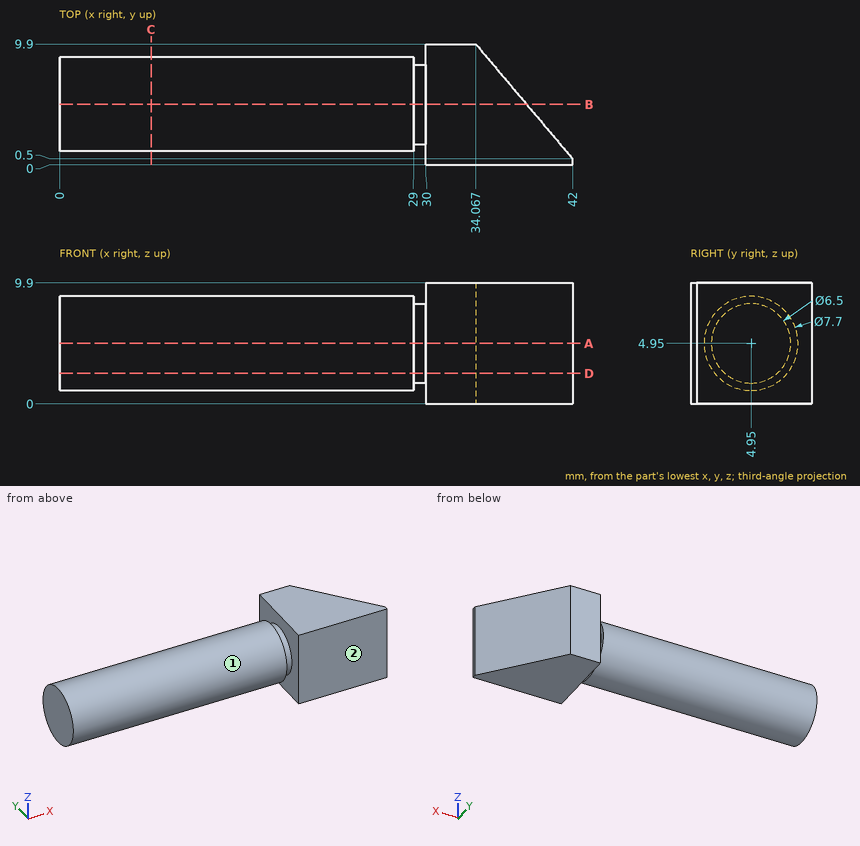
The drawing under review shows one solid part. Ordinate dimensions are in mm from its lowest x, y, z. A direction names the side the tool comes from. Give positions to 0.01 mm unless a question says otherwise; leave off trailing zeros. Write each loop counter-clockwise with the first axis right and the second up, starting at its lowest first coordinate (ties: lowest second). Pieces come first, ordered by that corner, then holes. Notation, with made-up numbers: (69.25, -2.5) - (126.25, -2.5) arc R21 cw to (126.25, 1.5) - close; hole circle Ø2 at (57, -3.5). An arc over 180 degrees is marked (long way). Answer in a Markdown table with one row per item. Add a question column.
1. Tool access review of the marked faces 1 and 2: name each direction out of +Z, -Z, +X, -X, +Y, -Y from which nothing blocks a thin tool from reaching the whole face with its end or side.
2. Wall thickness on line 1 along X through (y, z) = (0.5, 3.75); line 2 along Z through (x, y) = (6, 5): over which ranges is each line inside the solid? List them lowest first. Write a range as [from, to].
3. We need section A-A on z = 4.95. Write out the cut boundary in (x, y).
4. Insertion check: P1, Ø1.5, axis at x = 19.5, z = 2, coming from the -Y side; P2, Ø2, axis at y = 8, z = 7, coming from the +X side (1 decimal); P3, Ø1, axis at x = 16, y = 3, coming from the +Z side. Each pin has a flat end and moves straight along its axis. Give the tip position at first contact, or say it passes through.
5. We need section B-B on y = 4.95. Write out the cut boundary in (x, z).
6. We need section C-C on x = 7.5. Write out the cut boundary in (y, z), then the cut area to 3 significant figures.
7. We need section D-D on z = 2.5. Write out the cut boundary in (x, y), then the cut area to 3 significant figures.
Ans:
| question | item | result |
|---|---|---|
| 1 | face 1 | -X |
| 1 | face 2 | +Z, -Z, +X, -X, -Y |
| 2 | line 1 | x = [30, 42] |
| 2 | line 2 | z = [1.1, 8.8] |
| 3 | outline | (0, 1.1) - (29, 1.1) - (29, 1.7) - (30, 1.7) - (30, 0) - (42, 0) - (42, 0.5) - (34.07, 9.9) - (30, 9.9) - (30, 8.2) - (29, 8.2) - (29, 8.8) - (0, 8.8) - close |
| 4 | P1 | stops at y = 1.79 |
| 4 | P2 | stops at x = 36.5 |
| 4 | P3 | stops at z = 8.52 |
| 5 | outline | (0, 1.1) - (29, 1.1) - (29, 1.7) - (30, 1.7) - (30, 0) - (38.24, 0) - (38.24, 9.9) - (30, 9.9) - (30, 8.2) - (29, 8.2) - (29, 8.8) - (0, 8.8) - close |
| 6 | outline | circle Ø7.7 at (4.95, 4.95) |
| 6 | area | 46.6 mm^2 |
| 7 | outline | (0, 1.98) - (29, 1.98) - (29, 2.81) - (30, 2.81) - (30, 0) - (42, 0) - (42, 0.5) - (34.07, 9.9) - (30, 9.9) - (30, 7.09) - (29, 7.09) - (29, 7.92) - (0, 7.92) - close |
| 7 | area | 258 mm^2 |
